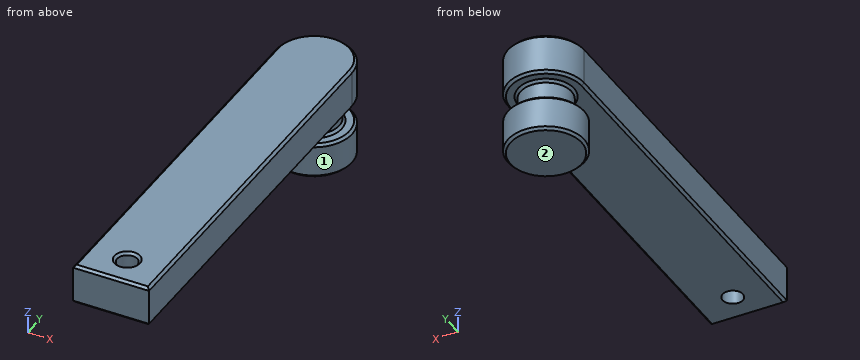
```python
from build123d import *

# Parameters (mm, degrees)
SKETCH3_R           = 2
BOSS_EXTRUDE1_DEPTH = 8
SKETCH4_R           = 5
BOSS_EXTRUDE2_DEPTH = 5
BOSS_EXTRUDE3_START = 7
SKETCH5_R           = 7.5
BOSS_EXTRUDE3_DEPTH = 7
CHAMFER1_SIZE       = 0.5


with BuildPart() as part:
    # Sketch3 → Boss-Extrude1 (new body)
    with BuildSketch(Plane.XY):
        with BuildLine():
            Line((7.5, 75), (7.5, 0))
            Line((7.5, 0), (-7.5, 0))
            Line((-7.5, 0), (-7.5, 75))
            ThreePointArc((-7.5, 75), (0, 82.5), (7.5, 75))
        make_face()
        with Locations((0, 6)):
            Circle(SKETCH3_R, mode=Mode.SUBTRACT)
    extrude(amount=BOSS_EXTRUDE1_DEPTH)

    # Sketch4 → Boss-Extrude2 (add)
    with BuildSketch(Plane.XY):
        with Locations((0, 75)):
            Circle(SKETCH4_R)
    extrude(amount=-BOSS_EXTRUDE2_DEPTH)

    # Sketch5 → Boss-Extrude3 (add)
    with BuildSketch(Plane(origin=(0, 0, -5), x_dir=(-1, 0, 0), z_dir=(0, 0, -1)).offset(BOSS_EXTRUDE3_START)):
        with Locations((0, 75)):
            Circle(SKETCH5_R)
    extrude(amount=-BOSS_EXTRUDE3_DEPTH)

    # Chamfer1
    chamfer1_edges = [part.edges().sort_by_distance(p)[0] for p in [
        (-2, 6, 8),
        (7.5, 37.5, 8),
        (0, 82.5, 8),
        (-5, 75, 0),
        (-5, 75, -5),
        (7.5, 75, -5),
        (7.5, 75, -12),
        (-7.5, 37.5, 8),
        (0, 82.5, 0),
        (7.5, 37.5, 0),
        (0, 0, 0),
        (-7.5, 37.5, 0),
        (0, 0, 8),
    ]]
    chamfer(chamfer1_edges, length=CHAMFER1_SIZE)


solid = part.part
```
Check sheet for the modelled part. Datum: model origin and axes. Units: mm. Face numbers are marked on the shaded views. A direction names the side the tool comes from. Give positions to 0.01 mm unless a question says otherwise; leave off trailing zeros. Loops run counter-clockwise (first coordinate to the right, second up) from the corner with the lowest first, then second, coordinate; pieces in that order, holes last. Notation, with made-up numbers: M 5,-18.5 L 41,-18.5 A18 ccw 41,-0.5 Z; hole C 51.5,-0.75 d9. An arc over 180 degrees is marked long. Answer as CSV lines item,"result".
Item 1: Set-up check for the marked faces 1 and 2: record each of +Z, -Z, +X, -X, +Y, -Y from which the full face is reachable in a straight line by a thin tool's end or side.
Reply:
face 1,"-Z"
face 2,"-Z, +X, -X, +Y, -Y"
Item 2: Sectioned sample at D-D, the plane y = 28.5. Enter the section's corners in (x, z), then the cut area to 4 significant figures.
Reply:
outline,"M -7.5,0.5 L -7,0 L 7,0 L 7.5,0.5 L 7.5,7.5 L 7,8 L -7,8 L -7.5,7.5 Z"
area,"119.5 mm^2"
Item 3: Depth check by flat-ended pin: pin 1 Ø8 at (x, z) = (-2, 2) entering from -Y; pin 2 Ø4 at (x, y) = (1.5, 52.5) entering from -Z; pin 3 Ø1.5 at (x, z) = (4, -2.5) entering from +Y; pin 4 Ø1 at (x, z) = (-3.5, 3) entering from +Y. Enter the tip coordinate at first touch or a pass-through.
Reply:
pin 1,"y = 0"
pin 2,"z = 0"
pin 3,"y = 78.8"
pin 4,"y = 81.87"
Item 4: Sectioned sample at A-A, the plane y = 6. Enter the section's corners in (x, z).
Reply:
outline,"M -7.5,0.5 L -7,0 L -2,0 L -2,7.5 L -2.5,8 L -7,8 L -7.5,7.5 Z; M 2,0 L 7,0 L 7.5,0.5 L 7.5,7.5 L 7,8 L 2.5,8 L 2,7.5 Z"
Item 5: Sectioned sample at C-C, the plane z = 2.5. Enter the section's corners in (x, y), then the cut area to 3 significant figures.
Reply:
outline,"M -7.5,0 L 7.5,0 L 7.5,75 A7.5 ccw -7.5,75 Z; hole C 0,6 d4"
area,"1,200 mm^2"
Item 6: Scan lines: L1, parallel to Z at x = 5.5, y = 77.5; L2, parallel to Y at x = 0, z = 2.5; L3, parallel to Z at x = 6.25, y = 23. Record each from-to range of solid material in increasing order.
Reply:
L1,"-12 to -5, 0 to 8"
L2,"0 to 4, 8 to 82.5"
L3,"0 to 8"
